For this review, take the finished solid that the model builds, in its own axes (mm). A direction names the side the tool comes from. Coordinates: 2 decimals unless noted, no trailing zeros. Write each loop counter-clockwise with the first axis right and the second up, starting at its lowest first coordinate (ties: lowest second). Pieces come first, ordered by that corner, then holes.
```python
from build123d import *

# Parameters (mm, degrees)
BOSS_EXTRUDE1_DEPTH = 43
SKETCH2_W           = 3.5
SKETCH2_H           = 2.25
CUT_EXTRUDE1_DEPTH  = 0.5
SKETCH3_W           = 4.15
SKETCH3_H           = 3.2
SKETCH3_W_2         = 3
CUT_EXTRUDE2_DEPTH  = 0.75
SKETCH5_R           = 1.25
CUT_EXTRUDE3_DEPTH  = 0.25
SKETCH6_W           = 1.326960347
SKETCH6_H           = 0.484850896
BOSS_EXTRUDE2_DEPTH = 0.25
SKETCH7_W           = 3.7
SKETCH7_H           = 2.8
CUT_EXTRUDE4_DEPTH  = 1.7


with BuildPart() as part:
    # Sketch1 → Boss-Extrude1 (new body)
    with BuildSketch(Plane(origin=(0, 0, 0), x_dir=(1, 0, 0), z_dir=(0, 1, 0))):
        with BuildLine():
            Line((-10.25, 4.5), (10.25, 4.5))
            ThreePointArc((10.25, 4.5), (14.75, 0), (10.25, -4.5))
            Line((10.25, -4.5), (-10.25, -4.5))
            ThreePointArc((-10.25, -4.5), (-14.75, 0), (-10.25, 4.5))
        make_face()
    extrude(amount=BOSS_EXTRUDE1_DEPTH)

    # Sketch2 → Cut-Extrude1 (cut)
    with BuildSketch(Plane(origin=(0, 43, 0), x_dir=(1, 0, 0), z_dir=(0, 1, 0))):
        with Locations((-10.319273123, -2.424555182)):
            Rectangle(SKETCH2_W, SKETCH2_H)
        Polygon((6.661858634, 0), (4.410192585, 1.3), (4.410192585, -1.3), align=None)
    extrude(amount=-CUT_EXTRUDE1_DEPTH, mode=Mode.SUBTRACT)

    # Sketch3 → Cut-Extrude2 (cut)
    with BuildSketch(Plane.XZ):
        with Locations((-9.075, -1.6)):
            Rectangle(SKETCH3_W, SKETCH3_H)
        with Locations((-4.2, -1.6)):
            Rectangle(SKETCH3_W_2, SKETCH3_H)
        with Locations((0.775, -1.6)):
            Rectangle(SKETCH3_W, SKETCH3_H)
        with Locations((5.35, -1.6)):
            Rectangle(SKETCH3_W_2, SKETCH3_H)
    extrude(amount=-CUT_EXTRUDE2_DEPTH, mode=Mode.SUBTRACT)

    # Sketch5 → Cut-Extrude3 (cut)
    with BuildSketch(Plane.XZ):
        with Locations((-9.075, 2.25)):
            Circle(SKETCH5_R)
        with Locations((-4.2, 2.25)):
            Circle(SKETCH5_R)
        with Locations((0.775, 2.25)):
            Circle(SKETCH5_R)
        with Locations((5.35, 2.25)):
            Circle(SKETCH5_R)
    extrude(amount=-CUT_EXTRUDE3_DEPTH, mode=Mode.SUBTRACT)

    # Sketch6 → Boss-Extrude2 (add)
    with BuildSketch(Plane.XZ.offset(-0.25)):
        Polygon((-9.319136071, 2.080501294), (-9.924638911, 2.080501294), (-9.924638911, 2.512434892), (-9.319136071, 2.512434892), (-9.319136071, 3.219423302), (-8.814550371, 3.219423302), (-8.814550371, 2.512434892), (-8.194630797, 2.512434892), (-8.194630797, 2.080501294), (-8.814550371, 2.080501294), (-8.814550371, 1.323622745), (-9.319136071, 1.323622745), align=None)
        with Locations((0.807600037, 2.270009444)):
            Rectangle(SKETCH6_W, SKETCH6_H)
        with BuildLine():
            Line((4.715564351, 1.80853907), (4.912980216, 1.997240994))
            add(Edge.make_bspline(
                [(4.912980216, 1.997240994), (4.929707146, 1.979899926), (4.962433267, 1.945972249), (5.015418116, 1.901557226), (5.069888716, 1.863810031), (5.125997527, 1.833043383), (5.183712319, 1.808626724), (5.243133504, 1.791593673), (5.30411755, 1.780868656), (5.345327837, 1.77968748), (5.366105216, 1.779091955)],
                knots=[0, 0, 0, 0, 7.224e-05, 0.000141338, 0.000207016, 0.000270758, 0.000332981, 0.000394603, 0.000455858, 0.000518145, 0.000518145, 0.000518145, 0.000518145], degree=3))
            add(Edge.make_bspline(
                [(5.366105216, 1.779091955), (5.383454547, 1.779571665), (5.417691539, 1.78051832), (5.467955666, 1.787474955), (5.516054131, 1.799260394), (5.562025094, 1.815642069), (5.60609584, 1.836272091), (5.647855993, 1.862202541), (5.687529977, 1.892567959), (5.724654232, 1.927315209), (5.758169405, 1.965560051), (5.788367052, 2.005838724), (5.813379552, 2.048863663), (5.833797229, 2.09400743), (5.849886827, 2.141286329), (5.86130626, 2.190697991), (5.867922688, 2.24235398), (5.868909154, 2.277470612), (5.869410505, 2.295317917)],
                knots=[0, 0, 0, 0, 5.2039e-05, 0.000102693, 0.000151885, 0.000200355, 0.000248878, 0.000297579, 0.000347521, 0.000398543, 0.000449848, 0.000499909, 0.000549331, 0.000598819, 0.000648325, 0.000698909, 0.000750715, 0.000804255, 0.000804255, 0.000804255, 0.000804255], degree=3))
            add(Edge.make_bspline(
                [(5.869410505, 2.295317917), (5.869263959, 2.307844037), (5.868975113, 2.332533276), (5.86589296, 2.368961679), (5.860774249, 2.404382271), (5.853594852, 2.438690106), (5.844556603, 2.472033181), (5.833494646, 2.504194313), (5.820119677, 2.535214768), (5.805150865, 2.565257037), (5.788442474, 2.594066561), (5.769713133, 2.621261294), (5.74917272, 2.646629922), (5.727643129, 2.671055186), (5.703698503, 2.693107682), (5.678410927, 2.714002754), (5.651417573, 2.733222757), (5.622751223, 2.750500219), (5.593267533, 2.766602513), (5.562362337, 2.779937286), (5.530899248, 2.791924454), (5.498326297, 2.800942411), (5.465217256, 2.808786127), (5.431111276, 2.813576528), (5.396332037, 2.8172166), (5.372826074, 2.817440712), (5.360997043, 2.817553494)],
                knots=[0, 0, 0, 0, 3.7571e-05, 7.4053e-05, 0.000109578, 0.000144878, 0.000179138, 0.000213158, 0.000246813, 0.000280408, 0.000313803, 0.000346642, 0.00037935, 0.000411691, 0.000444216, 0.00047688, 0.000510064, 0.000543509, 0.000577252, 0.000610751, 0.000644407, 0.00067817, 0.000712066, 0.000746402, 0.000781414, 0.000816882, 0.000816882, 0.000816882, 0.000816882], degree=3))
            add(Edge.make_bspline(
                [(5.360997043, 2.817553494), (5.340932624, 2.81697445), (5.301511258, 2.81583678), (5.24366326, 2.806901525), (5.188381183, 2.792269684), (5.144297695, 2.774670447), (5.109804461, 2.757561474), (5.083558758, 2.7419627), (5.056533291, 2.724293685), (5.028913098, 2.70406497), (5.000548666, 2.681517285), (4.971927273, 2.656179356), (4.94232014, 2.628879026), (4.922924645, 2.609394521), (4.912980216, 2.599404455)],
                knots=[0, 0, 0, 0, 6.0171e-05, 0.000118221, 0.000175146, 0.00023139, 0.000260282, 0.000290584, 0.000322921, 0.000357119, 0.000393253, 0.000431582, 0.000471767, 0.00051405, 0.00051405, 0.00051405, 0.00051405], degree=3))
            Line((4.912980216, 2.599404455), (4.721573966, 2.80042609))
            add(Edge.make_bspline(
                [(4.721573966, 2.80042609), (4.735028795, 2.813416305), (4.761289744, 2.838770428), (4.800903659, 2.874770908), (4.840467708, 2.907121373), (4.879026152, 2.936995856), (4.917210456, 2.963524548), (4.955017137, 2.98673217), (4.992016231, 3.00721189), (5.028982989, 3.024596757), (5.066210855, 3.039452525), (5.104498273, 3.051981146), (5.143863537, 3.062917773), (5.184632673, 3.071524335), (5.226623771, 3.078530672), (5.269971765, 3.083160305), (5.314474118, 3.086370664), (5.344564827, 3.086645271), (5.35979512, 3.086784263)],
                knots=[0, 0, 0, 0, 5.6107e-05, 0.000109509, 0.000160524, 0.000209386, 0.000255813, 0.000299927, 0.000342421, 0.000382612, 0.000422396, 0.000462589, 0.000503412, 0.000544902, 0.000587533, 0.000631069, 0.000675641, 0.000721323, 0.000721323, 0.000721323, 0.000721323], degree=3))
            add(Edge.make_bspline(
                [(5.35979512, 3.086784263), (5.387770205, 3.086069862), (5.44250967, 3.084671977), (5.522736662, 3.074350257), (5.599013379, 3.056931828), (5.671476881, 3.03263203), (5.739905397, 3.001078873), (5.804513521, 2.962792741), (5.865193661, 2.917410259), (5.921423669, 2.865607584), (5.972270451, 2.808383842), (6.017263923, 2.746964786), (6.05431883, 2.680909351), (6.085758013, 2.611632486), (6.109316906, 2.538051127), (6.126465703, 2.460830166), (6.136900657, 2.379638221), (6.138053378, 2.324195186), (6.138641274, 2.295918878)],
                knots=[0, 0, 0, 0, 8.3912e-05, 0.000164192, 0.000242185, 0.000318297, 0.000393051, 0.000467825, 0.000543186, 0.000619954, 0.000696787, 0.000772517, 0.000847877, 0.000923602, 0.00100038, 0.001079187, 0.001160659, 0.001245459, 0.001245459, 0.001245459, 0.001245459], degree=3))
            add(Edge.make_bspline(
                [(6.138641274, 2.295918878), (6.138384513, 2.277478096), (6.137875675, 2.240932973), (6.132859378, 2.186959442), (6.12516416, 2.134563275), (6.114212057, 2.083808916), (6.100594572, 2.034520629), (6.083261482, 1.986921578), (6.063185313, 1.940751187), (6.039746603, 1.896439727), (6.013473059, 1.853931201), (5.984748971, 1.813333056), (5.953021206, 1.775049105), (5.918591266, 1.738911903), (5.881745297, 1.704687885), (5.842122948, 1.672619943), (5.799686332, 1.642914873), (5.754868318, 1.615548264), (5.708522141, 1.590415811), (5.660614863, 1.569342312), (5.612080106, 1.550739522), (5.56258902, 1.535713643), (5.512032672, 1.524379585), (5.460797123, 1.51582654), (5.408463744, 1.51103959), (5.373325792, 1.51025649), (5.355588389, 1.509861186)],
                knots=[0, 0, 0, 0, 5.5309e-05, 0.000109609, 0.000162473, 0.0002141, 0.00026528, 0.000315751, 0.000365939, 0.000416209, 0.000465993, 0.000515768, 0.000565283, 0.000615018, 0.00066541, 0.000716045, 0.000767813, 0.000820688, 0.000873519, 0.000925843, 0.000977576, 0.001029382, 0.001080845, 0.001132911, 0.001185116, 0.001238332, 0.001238332, 0.001238332, 0.001238332], degree=3))
            add(Edge.make_bspline(
                [(5.355588389, 1.509861186), (5.340456681, 1.510088069), (5.310350592, 1.510539475), (5.265516337, 1.514295789), (5.221045554, 1.52021179), (5.177074042, 1.529075404), (5.133404064, 1.539809648), (5.090218454, 1.553031339), (5.047636298, 1.569158702), (5.005288443, 1.58699897), (4.964019452, 1.607309189), (4.924187982, 1.630042499), (4.885695338, 1.654604176), (4.848773565, 1.681416683), (4.813162609, 1.71008618), (4.778900466, 1.740611719), (4.746315906, 1.773547024), (4.72586669, 1.796816088), (4.715564351, 1.80853907)],
                knots=[0, 0, 0, 0, 4.5389e-05, 9.0305e-05, 0.000134883, 0.000179905, 0.000224797, 0.000269754, 0.000315297, 0.000361342, 0.000407569, 0.000453187, 0.000498865, 0.000544484, 0.000590004, 0.000635969, 0.000682075, 0.000728889, 0.000728889, 0.000728889, 0.000728889], degree=3))
        make_face()
        Polygon((-3.830473477, 1.548322724), (-4.638165785, 1.548322724), (-4.638165785, 1.817553494), (-4.368935016, 1.817553494), (-4.368935016, 3.048322724), (-4.099704247, 3.048322724), (-4.099704247, 1.817553494), (-3.830473477, 1.817553494), align=None)
    extrude(amount=BOSS_EXTRUDE2_DEPTH)

    # Sketch7 → Cut-Extrude4 (cut)
    with BuildSketch(Plane.XZ):
        with Locations((-12.9, 3.1)):
            Rectangle(SKETCH7_W, SKETCH7_H)
        with Locations((12.9, 3.1)):
            Rectangle(SKETCH7_W, SKETCH7_H)
    extrude(amount=-CUT_EXTRUDE4_DEPTH, mode=Mode.SUBTRACT)


solid = part.part
```
Q1. Tool access review of faces 5 (the flat face through (-12, 1.7, 3)), 6 (the flat face through (1, 0.75, -2)), 7 (the flat face through (11.05, 1, 3)): name each direction out of +Z, -Z, +X, -X, +Y, -Y from which nothing blocks a thin tool from reaching the whole face with its end or side.
Ans:
face 5: +Z, -X, -Y
face 6: -Y
face 7: +Z, +X, -Y
Q2. For probe 1 along Z at (x, y) = (-4.2, 0.15); probe 2 along Y at (x, z) = (5.25, -0.75); probe 3 along Y at (x, z) = (0, 2.25), list the stretches that pass through material, from the lowest coordinate up.
Ans:
probe 1: z = -4.5 to -3.2, 0 to 1, 1.55 to 3.05, 3.5 to 4.5
probe 2: y = 0.75 to 42.5
probe 3: y = 0.25 to 43
Q3. Add section A-A (y = 3.5). State the section outline as (x, z) points, then the cut area to 3 significant figures.
Ans:
outline: (-10.25, -4.5) - (10.25, -4.5) arc R4.5 ccw to (10.25, 4.5) - (-10.25, 4.5) arc R4.5 ccw to start
area: 248 mm2
Q4. Clearance check with flat-ended pins moving along their axes: pin 1 Ø0.9 at (x, z) = (5, -2) entering from -Y; pin 2 Ø0.6 at (y, z) = (0.5, -1.5) entering from +X; pin 3 Ø1.4 at (x, z) = (-12.5, 3) entering from -Y. State where each tip first meets the part, or that it passes through.
Ans:
pin 1: stops at y = 0.75
pin 2: stops at x = 14.59
pin 3: stops at y = 1.7
Q5. Add section B-B (z = -2). State the section outline as (x, y) points.
Ans:
outline: (-14.28, 0) - (-11.15, 0) - (-11.15, 0.75) - (-7, 0.75) - (-7, 0) - (-5.7, 0) - (-5.7, 0.75) - (-2.7, 0.75) - (-2.7, 0) - (-1.3, 0) - (-1.3, 0.75) - (2.85, 0.75) - (2.85, 0) - (3.85, 0) - (3.85, 0.75) - (6.85, 0.75) - (6.85, 0) - (14.28, 0) - (14.28, 43) - (-14.28, 43) - close
Q6. Draft analysis for pull direction Z (two halves, no side actions). For faces 1 (the flat face through (13, 1, 1.7)), 2 (the flat face through (5.3, 0.25, 2.3)), 3 (the flat face through (12, 1.7, 3)), 4 (the flat face through (5.52, 42.75, 0.66)), state which applies: +Z half, -Z half, draft (parallel to the pull), parting line (faces both ways), or undercut.
Ans:
face 1: +Z half
face 2: undercut
face 3: draft
face 4: undercut
